Verification items for the finished model (mm, model axes). Give positions to 0.01 mm unless a question says otherwise; leave off trailing zeros. Loops run counter-clockwise (first coordinate to the right, second up) from the corner with the lowest first, then second, coordinate; pieces in that order, holes last. Notation, with made-up numbers: (72.5, 48) -> (117.5, 48) arc R6 ccw to (117.5, 52) -> close; hole circle Ø3 at (1, 3). An arc over 180 degrees is marked (long way). Answer in a Markdown table with one row per item. Add a question column.
Q1. Gauge pin test, flat ends, axial feed: P1, Ø2, axis at x = -4, y = 49, coming from the +Z side; P2, Ø5, axis at x = -28.5, y = 44, coming from the +Z side; P3, Ø12, axis at y = 29.5, z = 44, coming from the -X side. Record the tip position at first contact, or that the pin passes through.
Q2. Section check B-B on z = 0. Enter the section's corners in (x, y), and give its area (3 significant figures).
Q3. Section check A-A on x = 0. Enter the section's corners in (y, z), and give its area (3 significant figures).
Q4. Material ranges on probe 1 along X at (y, z) = (51, 0); probe 2 along X at (y, z) = (7.5, 0); probe 3 along Z at (x, y) = (-14, 37.5), recorded low to high.
Q5. Section check C-C on y = 20. Enter the section's corners in (x, z).
```python
from build123d import *


with BuildPart() as part:
    # Szkic1 → Obrót1 (revolve)
    with BuildSketch(Plane.XY, mode=Mode.PRIVATE) as obr_t1_sk:
        Polygon((-65, 0), (-63, 0), (-63, 10), (-60, 10), (-60, 100), (-64, 100), (-64, 90), (-65, 90), (-65, 10), align=None)
    revolve(obr_t1_sk.sketch.rotate(Axis((0, 0, 0), (0, 1, 0)), 270), axis=Axis((0, 0, 0), (0, 1, 0)))


solid = part.part
```
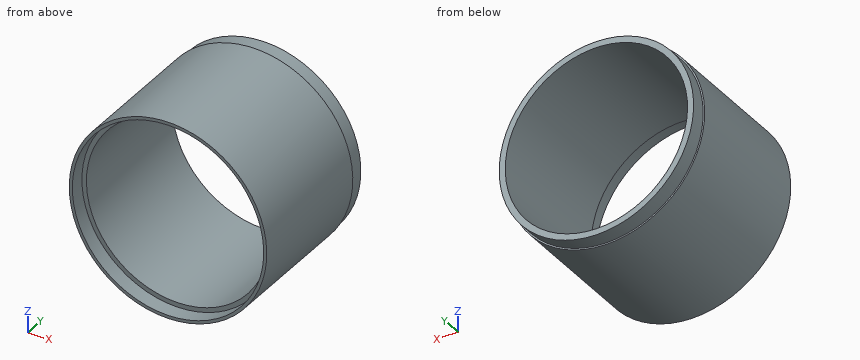
Taken from the geometry:
| question | item | result |
|---|---|---|
| 1 | P1 | stops at z = 64.93 |
| 1 | P2 | stops at z = 59.57 |
| 1 | P3 | stops at x = -52.74 |
| 2 | outline | (-65, 0) -> (-63, 0) -> (-63, 10) -> (-60, 10) -> (-60, 100) -> (-64, 100) -> (-64, 90) -> (-65, 90) -> close; (60, 10) -> (63, 10) -> (63, 0) -> (65, 0) -> (65, 90) -> (64, 90) -> (64, 100) -> (60, 100) -> close |
| 2 | area | 920 mm² |
| 3 | outline | (0, -65) -> (90, -65) -> (90, -64) -> (100, -64) -> (100, -60) -> (10, -60) -> (10, -63) -> (0, -63) -> close; (0, 63) -> (10, 63) -> (10, 60) -> (100, 60) -> (100, 64) -> (90, 64) -> (90, 65) -> (0, 65) -> close |
| 3 | area | 920 mm² |
| 4 | probe 1 | x = -65 to -60, 60 to 65 |
| 4 | probe 2 | x = -65 to -63, 63 to 65 |
| 4 | probe 3 | z = -63.47 to -58.34, 58.34 to 63.47 |
| 5 | outline | circle Ø130 at (0, 0); hole circle Ø120 at (0, 0) |
